Geometry: final body of the model. Coordinates: model frame, mm. Face numbers are marked on the shaded views. A direction names the side the tool comes from. Give positions to 0.01 mm unless a question says otherwise; leave off trailing zeros. Loops run counter-clockwise (first coordinate to the right, second up) from the corner with the lowest first, then second, coordinate; pieces in that order, holes last. Notation, with made-up numbers: M 60,73.5 L 119,73.5 A17 ccw 119,95.5 Z; hole C -0.75,-22.5 d9. An arc over 180 degrees is marked long. Put each result on its own line as item: value.
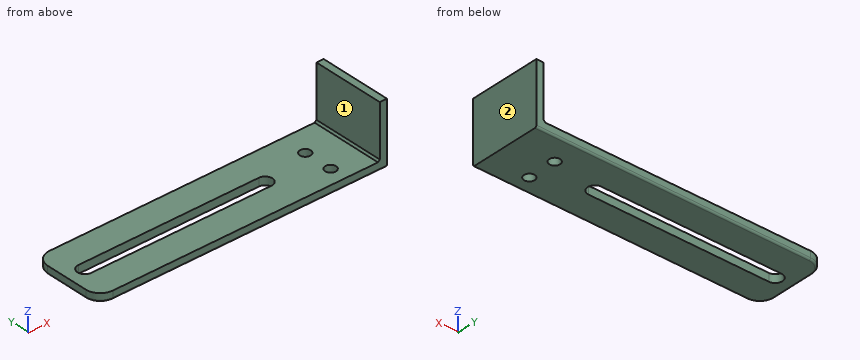
Autodesk Fusion 360 part; units mm, degrees
sketch "Sketch1" plane through (0, 0, 0) normal (0, 0, 1) x (1, 0, 0)
  line L0 (0, 0) -> (80, 0)
  line L1 (80, 0) -> (80, 20)
  line L2 (80, 20) -> (0, 20)
  line L3 (0, 20) -> (0, 0)
  line L4 (80, 20) -> (60, 20)
  line L5 (60, 20) -> (60, 0)
  line L6 (60, 0) -> (80, 0)
  line L7 (80, 0) -> (80, 20)
  line L8 (80, 20) -> (78, 20)
  line L9 (78, 20) -> (78, 0)
  line L10 (78, 0) -> (80, 0)
  line L11 (80, 0) -> (80, 20)
  line L12 (55, 12) -> (5, 12)
  arc A0 (5, 12) -> (5, 8) centre (5, 10) ccw
  line L13 (5, 8) -> (55, 8)
  arc A1 (55, 8) -> (55, 12) centre (55, 10) ccw
  line L14 (55, 10) -> (5, 10) construction
  point P0 (30, 10)
  dimension "d1" = 80
  dimension "d2" = 20
  dimension "d3" = 20
  dimension "d4" = 2
  dimension "d6" = 4
extrude "Extrude1" add sketch "Sketch1" along normal blind 2.2 contours L0 L2 L3 L5 | L0 L2 L4 L5 L6 L9
extrude "Extrude2" add sketch "Sketch1" along normal blind 15 contours L0 L1 L2 L4 L6 L7 L8 L9 L10 L11
chamfer "Chamfer1" distance 0.5 angle 45 1 edges at (78, 10, 2.2)
fillet "Fillet1" radius 4 2 edges at (0, 0, 1.1) (0, 20, 1.1)
fillet "Fillet2" radius 0.5 5 edges at (42, 20, 0) (1.1716, 18.8284, 0) (0, 10, 0) (1.1716, 1.1716, 0) (42, 0, 0)
sketch "Sketch2" plane through (0, 0, 2.2) normal (0, 0, 1) x (-1, 0, 0)
  arc A0 (-4, -20) -> (0, -16) centre (-4, -16) ccw
  line L0 (0, -16) -> (0, -4)
  arc A1 (0, -4) -> (-4, 0) centre (-4, -4) ccw
  line L1 (-4, 0) -> (-77.5, 0)
  line L2 (-77.5, 0) -> (-77.5, -20)
  line L3 (-77.5, -20) -> (-4, -20)
  arc A2 (-55, -8) -> (-55, -12) centre (-55, -10) ccw
  line L4 (-55, -8) -> (-5, -8)
  arc A3 (-5, -12) -> (-5, -8) centre (-5, -10) ccw
  line L5 (-5, -12) -> (-55, -12)
  line L6 (-77.5, 0) -> (-59.5, 0)
  line L7 (-59.5, 0) -> (-59.5, -20)
  line L8 (-59.5, -20) -> (-77.5, -20)
  line L9 (-77.5, -20) -> (-77.5, 0)
  circle A4 centre (-68.5, -4.7) radius 1.5
  circle A5 centre (-68.5, -12.7) radius 1.5
  dimension "d14" = 18
  dimension "d15" = 3
  dimension "d16" = 9
  dimension "d17" = 20
  dimension "d18" = 4.7
  dimension "d19" = 3
  dimension "d20" = 8
extrude "Extrude3" cut sketch "Sketch2" against normal blind 10 contours A4 | A5
extrude "Extrude4" add 1 faces at (78.6667, 13.3333, 15) along direction (0, 0, 1) blind 2
Item 1: Pin query (flat end, axial travel): pin 1 Ø4 at (x, z) = (57.5, 4) entering from +Y; pin 2 Ø8 at (x, y) = (49.5, 2.5) entering from +Z; pin 3 Ø2.5 at (x, y) = (68.5, 12.7) entering from +Z (3 decimals). Return the tip coordinate at first contact, or that it passes through.
Output values:
pin 1: y = 20
pin 2: z = 2.2
pin 3: through
Item 2: Set-up query: the marked faces 1 and 2. Return all of +Z, -Z, +X, -X, +Y, -Y with unobstructed straight access to the full face (end or side cutting, diameter ignored); none if empty.
Output values:
face 1: +Z, -X, +Y, -Y
face 2: +Z, -Z, +X, +Y, -Y
Item 3: Section D-D on z = 8. Output: boundary loops of the cut face in (x, y), then the cut area to 3 significant figures.
Output values:
outline: M 78,0 L 80,0 L 80,20 L 78,20 Z
area: 40.0 mm²
Item 4: Section C-C on x = 50. Output: boundary loops of the cut face in (y, z), then the cut area to 3 significant figures.
Output values:
outline: M 0,0.5 A0.5 ccw 0.5,0 L 8,0 L 8,2.2 L 0,2.2 Z; M 12,0 L 19.5,0 A0.5 ccw 20,0.5 L 20,2.2 L 12,2.2 Z
area: 35.1 mm²
Item 5: Section A-A on x = 68.5. Output: boundary loops of the cut face in (y, z).
Output values:
outline: M 0,0.5 A0.5 ccw 0.5,0 L 3.2,0 L 3.2,2.2 L 0,2.2 Z; M 6.2,0 L 11.2,0 L 11.2,2.2 L 6.2,2.2 Z; M 14.2,0 L 19.5,0 A0.5 ccw 20,0.5 L 20,2.2 L 14.2,2.2 Z
Item 6: Section B-B on y = 12.7. Output: boundary loops of the cut face in (x, z).
Output values:
outline: M 0,0.5 A0.5 ccw 0.5,0 L 67,0 L 67,2.2 L 0,2.2 Z; M 70,0 L 80,0 L 80,17 L 78,17 L 78,2.7 L 77.5,2.2 L 70,2.2 Z
Item 7: Line query: probe 1 along Y at (x, z) = (68.5, 1.65); probe 2 along X at (y, z) = (4.7, 0.5); probe 3 along Z at (x, y) = (49, 5). Output: solid intervals per line, ascending. Write a range as [from, to].
Output values:
probe 1: [0, 3.2], [6.2, 11.2], [14.2, 20]
probe 2: [0, 67], [70, 80]
probe 3: [0, 2.2]
